Input: part model. Units: mm. Frame: model coordinates. A direction names the side the tool comes from. Coordinates: 2 decimals unless noted, no trailing zeros. Loops run counter-clockwise (first coordinate to the right, second up) from the corner with the lowest first, then second, coordinate; pieces in that order, holes last. Notation, with made-up numbers: (-35, 2) -> (-7, 2) arc R26 ccw to (-7, 17) -> close; hole circle Ø5 at (5, -11.5). An arc over 180 degrees is marked (long way). Put each result on its own line as item: value. Start each with the question number.
1) Contact query for flat-ended pins moving along their axis: P1, Ø10, axis at y = -31, z = 1, coming from the -X side; P2, Ø1.5, axis at y = -32, z = -19.5, coming from the +X side (3 decimals); P3, Ø2, axis at x = 2.5, y = 4, coming from the -Z side. Output: stop coordinate, or through.
2) Cut plane C-C (x = 2.7). Return the cut outline in (y, z), plus the area to 3 significant figures.
3) Material intervals for L1, parallel to X at y = -33.5, z = 13 (3 decimals); L2, parallel to Z at x = 2.9, y = -0.5; L3, parallel to Y at x = 0.3, z = -21, sorted ascending.
4) Cut plane A-A (y = 0). Return the cut outline in (x, z) (3 decimals), plus the area to 3 significant figures.
5) Set-up query: faces 1 (the cylindrical face through (2.513, -28.798, -0.936)), 2 (the flat face through (4.445, 0, -28)). Return all of +Z, -Z, +X, -X, +Y, -Y with unobstructed straight access to the full face (end or side cutting, diameter ignored); none if empty.
6) Pull-direction query (Y, two-part tool) for faces 3 (the flat face through (4.445, 28, 0)), 4 (the cylindrical face through (2.51, -0.06, 26.67)), 5 (the cylindrical face through (2.51, 26.68, -0.17)); classes: pulls with the +Y half, pulls with the -Y half, needs draft (parallel to the pull), parting line crosses it, or undercut.
from build123d import *

# Parameters (mm, degrees)
SKETCH1_R           = 44.45
BOSS_EXTRUDE1_DEPTH = 0.635
SKETCH2_R           = 1.27
BOSS_EXTRUDE2_DEPTH = 3.81
CUT_EXTRUDE1_REACH  = 64.977
SKETCH3_R           = 25.4
FILLET1_R           = 1.27


with BuildPart() as part:
    # Sketch1 → Boss-Extrude1 (new body)
    with BuildSketch(Plane(origin=(0, 0, 0), x_dir=(0, 0, -1), z_dir=(1, 0, 0))):
        Circle(SKETCH1_R)
    extrude(amount=BOSS_EXTRUDE1_DEPTH)

    # Sketch2 → Boss-Extrude2 (add)
    with BuildSketch(Plane(origin=(0.635, 0, 0), x_dir=(0, 0, -1), z_dir=(1, 0, 0))):
        with Locations(Location((0, 27.94, 0), (0, 0, 180))):
            Circle(SKETCH2_R)
        with Locations(Location((27.94, 0, 0), (0, 0, 180))):
            Circle(SKETCH2_R)
        with Locations(Location((0, -27.94, 0), (0, 0, 180))):
            Circle(SKETCH2_R)
        with Locations(Location((-27.94, 0, 0), (0, 0, 180))):
            Circle(SKETCH2_R)
    extrude(amount=BOSS_EXTRUDE2_DEPTH)

    # Sketch3 → Cut-Extrude1 (cut, up to next)
    with BuildSketch(Plane(origin=(0.635, 0, 0), x_dir=(0, 0, -1), z_dir=(1, 0, 0)), mode=Mode.PRIVATE) as cut_extrude1_sk1:
        Circle(SKETCH3_R)
    cut_extrude1_tool1 = extrude(cut_extrude1_sk1.sketch, amount=-CUT_EXTRUDE1_REACH, mode=Mode.PRIVATE) & part.part
    add(cut_extrude1_tool1.solids().sort_by_distance((0.635, 0, 0))[0], mode=Mode.SUBTRACT)

    # Fillet1
    # the kernel refuses this fillet: 1.27 mm, written as the material it takes off along each edge
    with BuildSketch(Plane(origin=(0, 0, 0), x_dir=(0, 0, -1), z_dir=(0, -1, 0))) as fillet1_piece_1:
        with BuildLine():
            CenterArc((43.350147737, 1.27), FILLET1_R, 270, 60)
            Line((43.350147737, 0), (43.350147737, -0.0254))
            Line((43.350147737, -0.0254), (44.45, -0.0254))
            Line((44.45, -0.0254), (44.4754, 0))
            ThreePointArc((44.4754, 0), (44.4754, 0.3175), (44.471997045, 0.6223))
            Line((44.471997045, 0.6223), (44.45, 0.635))
        make_face()
    revolve(axis=Axis((0, 0, 0), (1, 0, 0)), mode=Mode.SUBTRACT)


solid = part.part
Results found:
1. P1: stops at x = 0
1. P2: stops at x = 0.635
1. P3: passes through
2. outline: circle Ø2.54 at (-27.94, 0); circle Ø2.54 at (0, -27.94); circle Ø2.54 at (0, 27.94); circle Ø2.54 at (27.94, 0)
2. area: 20.3 mm2
3. L1: x = 0 to 0.635
3. L2: z = -29.11 to -26.77, 26.77 to 29.11
3. L3: y = -38.86 to -14.29, 14.29 to 38.86
4. outline: (0, -43.35) arc R1.27 ccw to (0.635, -44.45) -> (0.635, -29.21) -> (4.445, -29.21) -> (4.445, -26.67) -> (0.635, -26.67) -> (0.635, -25.4) -> (0, -25.4) -> close; (0, 25.4) -> (0.635, 25.4) -> (0.635, 26.67) -> (4.445, 26.67) -> (4.445, 29.21) -> (0.635, 29.21) -> (0.635, 44.45) arc R1.27 ccw to (0, 43.35) -> close
4. area: 43.1 mm2
5. face 1: +X
5. face 2: +Z, -Z, +X, +Y, -Y
6. face 3: needs draft
6. face 4: parting line crosses it
6. face 5: undercut
